Autodesk Inventor part; units mm, degrees
ref_plane "YZ Plane" through (0, 0, 0) normal (1, 0, 0) x (0, 1, 0)
ref_plane "XZ Plane" through (0, 0, 0) normal (0, 1, 0) x (-1, 0, 0)
ref_plane "XY Plane" through (0, 0, 0) normal (0, 0, 1) x (1, 0, 0)
ref_plane "Work Plane1" through (0, 0, 0) normal (0, 0, 1) x (1, 0, 0)
sketch "Sketch1" plane through (0, 0, 0) normal (0, 0, 1) x (1, 0, 0)
  line L0 (24.13, -1.27) -> (20.32, -1.27)
  line L1 (20.32, -1.27) -> (20.32, 2.54)
  line L2 (20.32, 2.54) -> (24.13, 2.54)
  line L3 (24.13, 2.54) -> (24.13, -1.27)
  line L4 (-1.905, -1.27) -> (-1.905, 2.54)
  line L5 (-1.905, 2.54) -> (1.905, 2.54)
  line L6 (1.905, 2.54) -> (1.905, -1.27)
  line L7 (1.905, -1.27) -> (-1.905, -1.27)
  line L8 (-20.32, 2.54) -> (-20.32, -1.27)
  line L9 (-20.32, -1.27) -> (-24.13, -1.27)
  line L10 (-24.13, -1.27) -> (-24.13, 2.54)
  line L11 (-24.13, 2.54) -> (-20.32, 2.54)
  line L12 (-25.4, 3.81) -> (25.4, 3.81)
  line L13 (-25.4, -3.81) -> (-25.4, 3.81)
  line L14 (25.4, -3.81) -> (-25.4, -3.81)
  line L15 (25.4, 3.81) -> (25.4, -3.81)
  point P0 (0, 0)
extrude "Extrusion1" add sketch "Sketch1" against normal blind 19.05 contours L0 L1 L2 L3 | L4 L5 L6 L7 | L8 L9 L10 L11
sketch "Sketch2" plane through (-24.13, 2.54, 0) normal (0, 1, 0) x (1, 0, 0)
  line L0 (47.3075, 11.1125) -> (45.4025, 11.1125)
  line L1 (45.4025, 11.1125) -> (45.4025, 13.0175)
  line L2 (45.4025, 13.0175) -> (47.3075, 13.0175)
  line L3 (47.3075, 13.0175) -> (47.3075, 11.1125)
  line L4 (23.1775, 13.0175) -> (25.0825, 13.0175)
  line L5 (25.0825, 13.0175) -> (25.0825, 11.1125)
  line L6 (25.0825, 11.1125) -> (23.1775, 11.1125)
  line L7 (23.1775, 11.1125) -> (23.1775, 13.0175)
  line L8 (0.9525, 13.0175) -> (2.8575, 13.0175)
  line L9 (2.8575, 13.0175) -> (2.8575, 11.1125)
  line L10 (2.8575, 11.1125) -> (0.9525, 11.1125)
  line L11 (0.9525, 11.1125) -> (0.9525, 13.0175)
  point P0 (24.13, 0)
extrude "Extrusion2" cut sketch "Sketch2" against normal blind 3.81
ref_plane "Work Plane2" through (0, 0, 0) normal (0, 0, 1) x (1, 0, 0)
sketch "Sketch3" plane through (0, 0, 0) normal (0, 0, 1) x (1, 0, 0)
  line L0 (24.13, -1.27) -> (20.32, -1.27)
  line L1 (20.32, -1.27) -> (20.32, 2.54)
  line L2 (20.32, 2.54) -> (24.13, 2.54)
  line L3 (24.13, 2.54) -> (24.13, -1.27)
  line L4 (-1.905, -1.27) -> (-1.905, 2.54)
  line L5 (-1.905, 2.54) -> (1.905, 2.54)
  line L6 (1.905, 2.54) -> (1.905, -1.27)
  line L7 (1.905, -1.27) -> (-1.905, -1.27)
  line L8 (-20.32, 2.54) -> (-20.32, -1.27)
  line L9 (-20.32, -1.27) -> (-24.13, -1.27)
  line L10 (-24.13, -1.27) -> (-24.13, 2.54)
  line L11 (-24.13, 2.54) -> (-20.32, 2.54)
  line L12 (-25.4, 3.81) -> (25.4, 3.81)
  line L13 (-25.4, -3.81) -> (-25.4, 3.81)
  line L14 (25.4, -3.81) -> (-25.4, -3.81)
  line L15 (25.4, 3.81) -> (25.4, -3.81)
  point P0 (0, 0)
extrude "Extrusion3" add sketch "Sketch3" along normal blind 50.8 contours L0 L1 L2 L3 | L4 L5 L6 L7 | L8 L9 L10 L11 | L12 L15 L14 L13
sketch "Sketch4" plane through (-25.4, 3.81, 0) normal (0, 1, 0) x (1, 0, 0)
  circle A0 centre (12.377, -37.1786) radius 7.95
  circle A1 centre (37.977, -37.1786) radius 7.95
  line L0 (50.8, -50.8) -> (0, -50.8)
  point P0 (25.4, 0)
  dimension "d6" = 15.9
  dimension "d7" = 15.9
  dimension "d8" = 13.6214
extrude "Extrusion4" cut sketch "Sketch4" against normal blind 7.62
fillet "Fillet1" radius 3.175 2 edges at (-25.4, 0, 50.8) (25.4, 0, 50.8)
properties part number "Ultrasonic Mount_3DPrint"
Part model, mm, in its own coordinate system. A direction names the side the tool comes from. Round coordinates to 2 decimals unless told otherwise and drop trailing zeros. Write each loop counter-clockwise with the first axis right and the second up, starting at its lowest first coordinate (ties: lowest second). Pieces come first, ordered by that corner, then holes. Notation, with made-up numbers: M 2.25,13 L 14.25,13 A7 cw 14.25,23 Z; hole C 29,21.5 d9. An arc over 180 degrees is marked long. One line per question, with ' | ' between items.
(1) Saw through at C-C on y = -0.25. Count the separate pieces of the cut face and the enclosed holes in it, then the cut area to 3 significant figures.
Answer key:
separate pieces: 1 | enclosed holes: 5 | area: 2,390 mm^2
(2) Two-plate mould, pull along X, no slides. Class faces 1 (the face through (0, 1, -11.112)), 2 (the face through (25.4, 0, 23)), 3 (the face through (0, 3.81, 25)): released by +X, released by -X, zero draft, split by the parting line, or undercut.
Answer key:
face 1: undercut | face 2: released by +X | face 3: zero draft
(3) Probe line 1 along X through (y, z) = (2.25, -2.5) (3 decimals); line 2 along X through (y, z) = (-3.5, 36.5); line 3 along Z through (x, y) = (4.5, 3). List the from-to ranges inside material, lowest first.
Answer key:
line 1: x = -24.13 to -20.32, -1.905 to 1.905, 20.32 to 24.13 | line 2: x = -25.4 to -20.94, -5.1 to 4.66, 20.5 to 25.4 | line 3: z = 0 to 50.8
(4) 3-axis set-ups, long thin cutter, end or side, ignore diameter. For faces 4 (the face through (1.905, 1, -9)), 5 (the face through (-22, -1.27, -9)), 6 (the face through (22, 1, -13.018)): which of +Z, -Z, +X, -X, +Y, -Y reach the whole face in a straight line?
Answer key:
face 4: -Z, +Y, -Y | face 5: -Z, +X, -X, -Y | face 6: +Y, -Y
(5) Saw through at B-B on z = 41. Write the cut outline in (x, y).
Answer key:
outline: M -25.4,-3.81 L -19.99,-3.81 L -19.99,3.81 L -25.4,3.81 Z; M -6.05,-3.81 L 5.61,-3.81 L 5.61,3.81 L -6.05,3.81 Z; M 19.55,-3.81 L 25.4,-3.81 L 25.4,3.81 L 19.55,3.81 Z
(6) Saw through at A-A on x = -17. Write the cut outline in (y, z).
Answer key:
outline: M -3.81,0 L 3.81,0 L 3.81,30.29 L -3.81,30.29 Z; M -3.81,44.06 L 3.81,44.06 L 3.81,50.8 L -3.81,50.8 Z
(7) Pin check, flat tips, straight feed: pin 1 (4 mm diameter, centred on y = -1.5, z = -10.5, fed in from +X); pin 2 (1.9 mm diameter, centred on x = -23, z = -5, fed in from +Y); pin 3 (4 mm diameter, centred on y = 3, z = -4, fed in from -X); pin 4 (9.5 mm diameter, centred on x = -13.02, z = 37.18, fed in from +Y). Stop position of each tip, or through.
Answer key:
pin 1: stops at x = 24.13 | pin 2: stops at y = 2.54 | pin 3: stops at x = -24.13 | pin 4: passes through
(8) Saw through at D-D on x = 6. Write the cut outline in (y, z), then the cut area to 3 significant figures.
Answer key:
outline: M -3.81,0 L 3.81,0 L 3.81,32.71 L -3.81,32.71 Z; M -3.81,41.64 L 3.81,41.64 L 3.81,50.8 L -3.81,50.8 Z | area: 319 mm^2
